Answer from the drawing. Dimensions are ordinates in mm from the lowest x, y and z of the part. Give positions to 0.01 mm unless a question says otherwise; leave off trailing zeros. Order: outer loops, then holes, each group sorted by start corner. A loop starts at its lowest first (then second) coordinate and runs counter-clockwise, first axis right, second up.
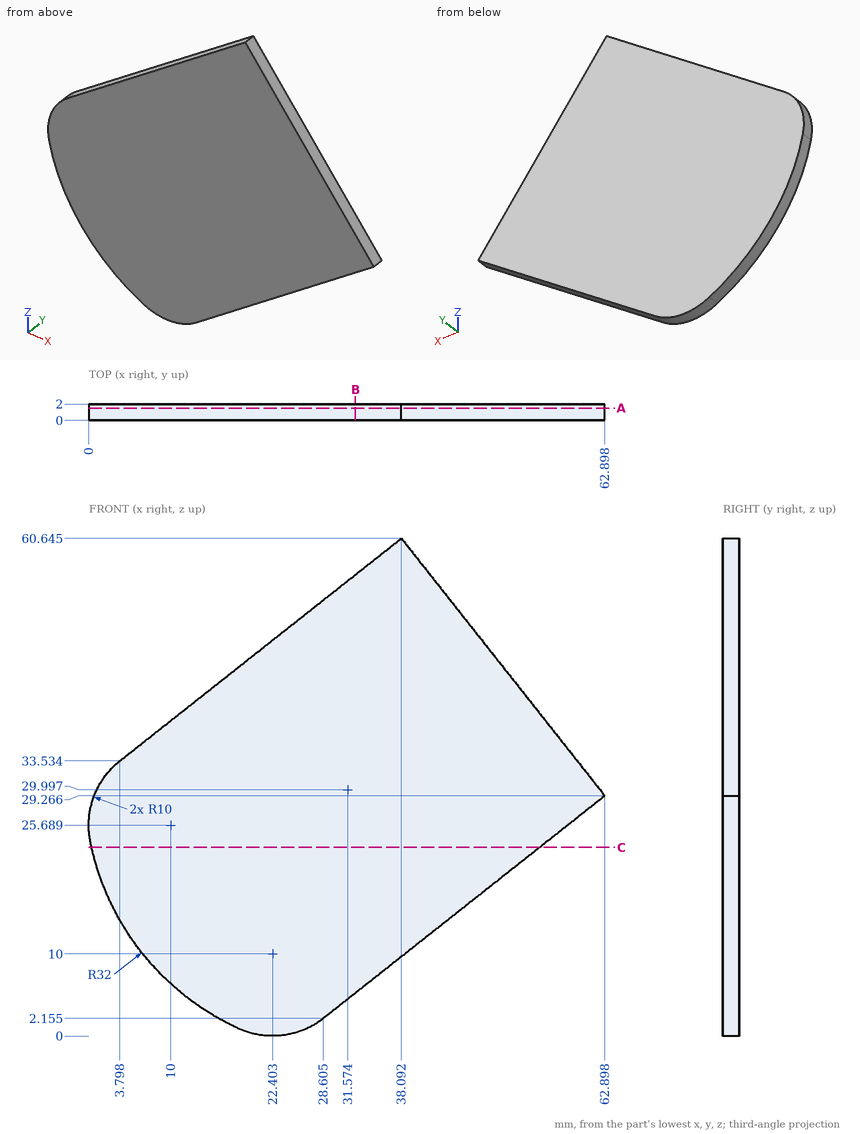
1. The part is cut by section A-A (y = 1.5). Write down the section's boundary in (x, z) (1 decimal), then the cut area to 3 significant figures.
Findings below:
outline: (0.2, 23.7) arc R32 ccw to (18.2, 0.9) arc R10 ccw to (28.6, 2.2) - (62.9, 29.3) - (38.1, 60.6) - (3.8, 33.5) arc R10 ccw to start
area: 2,150 mm2
2. Straight lines are drawn through the part: probe 1 along Z at (x, y) = (49.5, 1.3) (1 decimal); probe 2 along X at (y, z) = (1.3, 5.5) (1 decimal); probe 3 along Z at (x, y) = (24, 1.4) (1 decimal). For each, find the intervals that lie inside material, in ascending order.
Findings below:
probe 1: z = 18.7 to 46.2
probe 2: x = 11 to 32.8
probe 3: z = 0.1 to 49.5
3. Given P1, Ø8, axis at x = 44.5, z = 11, coming from the -Y side; P2, Ø1, axis at y = 0.5, z = 45.5, coming from the +X side, each flat-ended and moving along its own axis, determine where each tip first touches the part or whether it passes through.
Findings below:
P1: stops at y = 0
P2: stops at x = 50.46
4. The part is cut by section B-B (x = 32.5). Write down the section's boundary in (y, z) (1 decimal), then the cut area to 3 significant figures.
Findings below:
outline: (0, 5.2) - (2, 5.2) - (2, 56.2) - (0, 56.2) - close
area: 102 mm2
5. The part is cut by section C-C (z = 23). Write down the section's boundary in (x, y).
Findings below:
outline: (0.35, 0) - (54.97, 0) - (54.97, 2) - (0.35, 2) - close
